Answer from the drawing. Dimensions are ordinates in mm from the lowest x, y and z of the part. Coordinates: 2 decimals unless noted, no trailing zeros. Write each loop counter-clockwise with the first axis right and the second up, starting at its lowest first coordinate (ties: lowest second). Pieces come first, ordered by that corner, then holes.
(1) Straight lines are drawn through the part: line 1 along X through (y, z) = (33.5, 0.6); line 2 along Y through (x, z) = (30, 0.4); line 3 along X through (y, z) = (50, 1.3). For each, find the intervals that lie inside material, in ascending order.
(2) The part is cut by section A-A, the plane y = 47. Determine the outline of the cut face in (x, z), and give its area (3 significant figures).
(3) The part is cut by section C-C, the plane z = 0.3. Determine the outline of the cut face in (x, y), and give its area (3 significant figures).
(4) The part is cut by section B-B, the plane x = 30. Determine the outline of the cut face in (y, z).
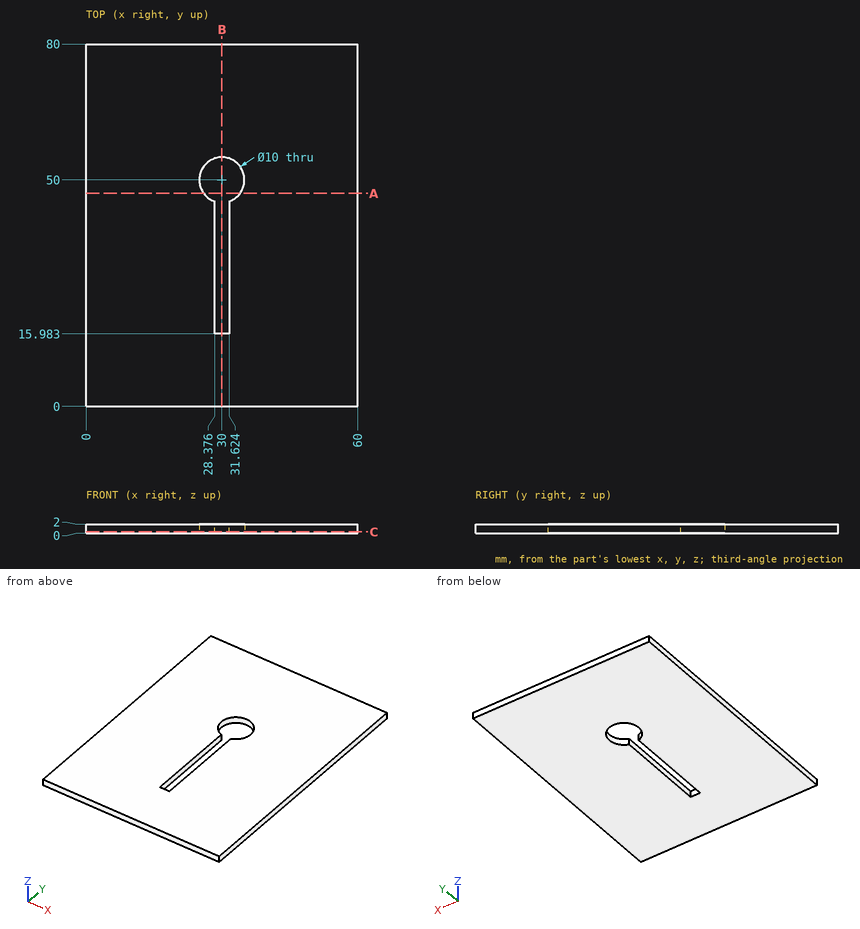
Computed:
1. line 1: x = 0 to 28.38, 31.62 to 60
1. line 2: y = 0 to 15.98, 55 to 80
1. line 3: x = 0 to 25, 35 to 60
2. outline: (0, 0) - (26, 0) - (26, 2) - (0, 2) - close; (34, 0) - (60, 0) - (60, 2) - (34, 2) - close
2. area: 104 mm2
3. outline: (0, 0) - (60, 0) - (60, 80) - (0, 80) - close; hole (28.38, 15.98) - (31.62, 15.98) - (31.62, 45.27) arc R5 ccw (long way) to (28.38, 45.27) - close
3. area: 4,630 mm2
4. outline: (0, 0) - (15.98, 0) - (15.98, 2) - (0, 2) - close; (55, 0) - (80, 0) - (80, 2) - (55, 2) - close
